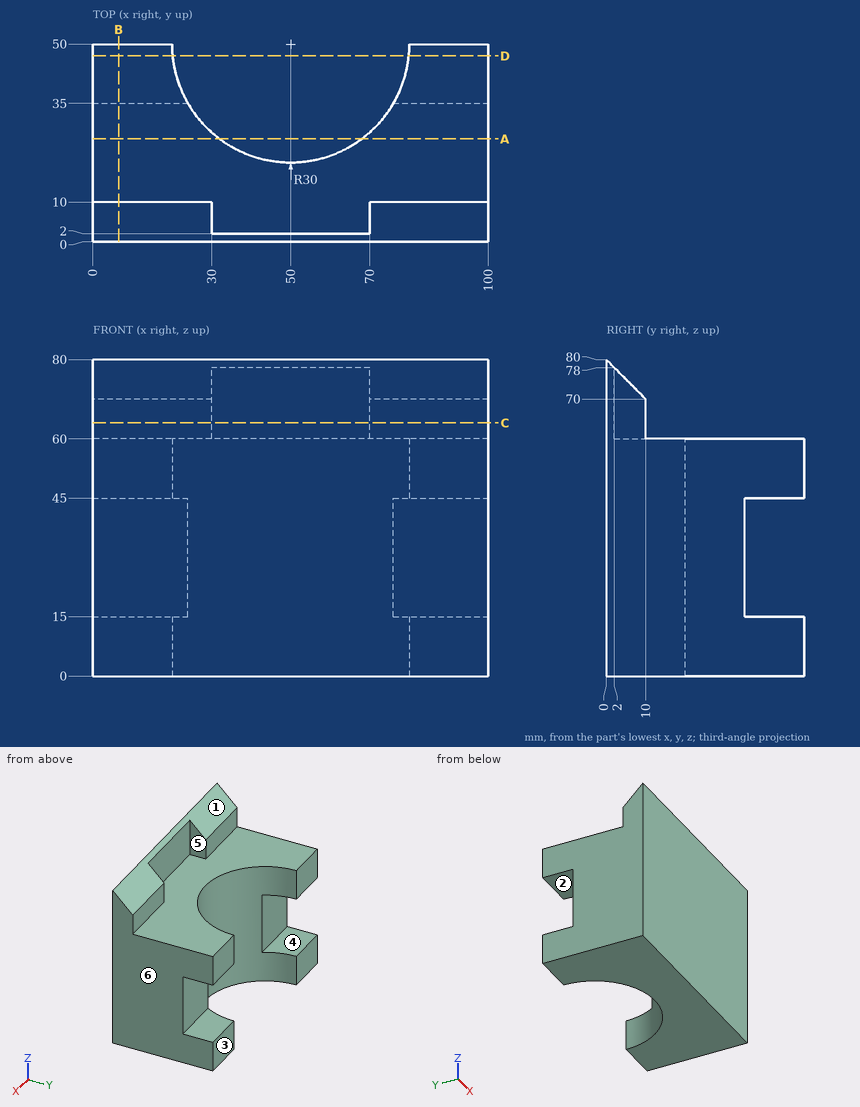
Job drawing, mm, ordinate dimensions from the low corner. One solid piece. A direction names the side the tool comes from. Give positions to 0.01 mm unless a question says otherwise; leave off trailing zeros. Order: outer loops, then holes, each group sorted by start corner. A loop starts at its lowest first (then second) coordinate and runs counter-clockwise, first axis right, second up. Notation, with made-up numbers: M 84,41 L 92,41 A36 cw 92,77 Z; hole C 13.5,20.5 d6. An arc over 180 degrees is marked long. Return JSON: item names as keys, results as strings.
Q1. Two-plate mould, pull along Z, no slides. Class the marked faces 1, 2 and 3: pulls with the +Z half, pulls with the -Z half, needs draft (parallel to the pull), parting line crosses it, or undercut.
Answer list:
{"face 1": "pulls with the +Z half", "face 2": "undercut", "face 3": "needs draft"}
Q2. Wall check: probe 1 along X at (y, z) = (6, 70); probe 2 along X at (y, z) = (26, 13.5); probe 3 along Z at (x, y) = (89.5, 37). Give the ranges that are in metal, low to high. Write a range as from..to.
Answer list:
{"probe 1": "x = 0..30, 70..100", "probe 2": "x = 0..32, 68..100", "probe 3": "z = 0..15, 45..60"}
Q3. Flat gauge pins, fed straight in: pin 1 (4.5 mm diameter, centred on x = 7, y = 46, fed in from -Z); pin 2 (4 mm diameter, centred on x = 80.5, y = 16, fed in from +Z); pin 3 (8 mm diameter, centred on x = 13.5, z = 66.5, fed in from +Y); pin 4 (8 mm diameter, centred on x = 83, z = 25.5, fed in from +Y). Where does each tip first touch, or does it go through?
Answer list:
{"pin 1": "stops at z = 0", "pin 2": "stops at z = 60", "pin 3": "stops at y = 10", "pin 4": "stops at y = 35"}
Q4. Band-saw the part on D-D (y = 47). Give the cut face in (x, z), then the cut area to 3 significant figures.
Answer list:
{"outline": "M 0,0 L 20.15,0 L 20.15,15 L 0,15 Z; M 0,45 L 20.15,45 L 20.15,60 L 0,60 Z; M 79.85,0 L 100,0 L 100,15 L 79.85,15 Z; M 79.85,45 L 100,45 L 100,60 L 79.85,60 Z", "area": "1,210 mm^2"}
Q5. Band-saw the part on A-A (y = 26). Give the cut face in (x, z), then the cut area to 3 significant figures.
Answer list:
{"outline": "M 0,0 L 32,0 L 32,60 L 0,60 Z; M 68,0 L 100,0 L 100,60 L 68,60 Z", "area": "3,840 mm^2"}
Q6. Band-saw the part on B-B (x = 6.5). Give the cut face in (y, z), then the cut area to 3 significant figures.
Answer list:
{"outline": "M 0,0 L 50,0 L 50,15 L 35,15 L 35,45 L 50,45 L 50,60 L 10,60 L 10,70 L 0,80 Z", "area": "2,700 mm^2"}
Q7. 3-axis set-ups, long thin cutter, end or side, ignore diameter. For the marked faces 4, 5 and 6: which of +Z, -Z, +X, -X, +Y, -Y reach the whole face in a straight line?
Answer list:
{"face 4": "+X, -X, +Y", "face 5": "+Z, +Y", "face 6": "+Z, -Z, +X, +Y, -Y"}
Q8. Band-saw the part on C-C (z = 64). Give the cut face in (x, y), then the cut area to 3 significant figures.
Answer list:
{"outline": "M 0,0 L 100,0 L 100,10 L 70,10 L 70,2 L 30,2 L 30,10 L 0,10 Z", "area": "680 mm^2"}
